```python
from build123d import *

# Parameters (mm, degrees)
ESBO_O1_R                = 5.857023813
RESSALTO_EXTRUS_O1_DEPTH = 2


with BuildPart() as part:
    # Esboço1 → Ressalto-extrusão1 (new body)
    with BuildSketch(Plane(origin=(0, 0, 0), x_dir=(1, 0, 0), z_dir=(0, 1, 0))):
        Polygon((-20, 48), (-39, 30), (-39, -30), (39, -30), (39, 30), (20, 48), align=None)
        with Locations(Location((-20, -15.384615385, 0), (0, 0, 270))):
            Circle(ESBO_O1_R, mode=Mode.SUBTRACT)
        with Locations(Location((20, -15.384615385, 0), (0, 0, 90))):
            Circle(ESBO_O1_R, mode=Mode.SUBTRACT)
    extrude(amount=RESSALTO_EXTRUS_O1_DEPTH)


solid = part.part
```
Geometry: final body of the model. Coordinates: model frame, mm. Round coordinates to 2 decimals unless told otherwise and drop trailing zeros. Loops run counter-clockwise (first coordinate to the right, second up) from the corner with the lowest first, then second, coordinate; pieces in that order, holes last. Notation, with made-up numbers: (42.25, 46.25) -> (79.25, 46.25) arc R19 ccw to (79.25, 72.25) -> close; hole circle Ø5 at (-35.75, -38.5). An arc over 180 degrees is marked (long way). Write each question's results on one line, items separated by ' | '.
Item 1: Pull-direction query (Z, two-part tool) for faces 1 (the face through (0, 1, -48)), 2 (the face through (39, 1, 0)), 3 (the face through (23.564, 0.986, 20.033)); classes: pulls with the +Z half, pulls with the -Z half, needs draft (parallel to the pull), parting line crosses it, or undercut.
Answers below:
face 1: pulls with the -Z half | face 2: needs draft | face 3: undercut
Item 2: Cut plane C-C on x = 34. Return the cut outline in (y, z).
Answers below:
outline: (0, -34.74) -> (2, -34.74) -> (2, 30) -> (0, 30) -> close
Item 3: Cut plane B-B on z = -40.5. Return the cut outline in (x, y), and give its area (3 significant figures).
Answers below:
outline: (-27.92, 0) -> (27.92, 0) -> (27.92, 2) -> (-27.92, 2) -> close | area: 112 mm²
Item 4: Pin query (flat end, axial travel): pin 1 Ø10.5 at (x, z) = (-20, 15.38) entering from +Y. Return the tip coordinate at first contact, or that it passes through.
Answers below:
pin 1: passes through
Item 5: Line query: probe 1 along Z at (x, y) = (20, 1.3); probe 2 along X at (y, z) = (0.6, 17); probe 3 along X at (y, z) = (0.15, 19.5). Output: solid intervals per line, ascending. Write a range as [from, to].
Answers below:
probe 1: z = [-48, 9.53], [21.24, 30] | probe 2: x = [-39, -25.63], [-14.37, 14.37], [25.63, 39] | probe 3: x = [-39, -24.17], [-15.83, 15.83], [24.17, 39]
Item 6: Cut plane A-A on y = 1.65. Return the cut outline in (x, z).
Answers below:
outline: (-39, -30) -> (-20, -48) -> (20, -48) -> (39, -30) -> (39, 30) -> (-39, 30) -> close; hole circle Ø11.71 at (-20, 15.38); hole circle Ø11.71 at (20, 15.38)
